from build123d import *

# Parameters (mm, degrees)
F0_W     = 16
F0_H     = 34
F1_DEPTH = 16
F2_W     = 10
F2_H     = 10
F3_DEPTH = 30
F4_W     = 10
F4_H     = 10
F5_DEPTH = 30
F6_R     = 1.5
F7_DEPTH = 16


with BuildPart() as f1:
    # F0 (on Top) → F1 (new body)
    with BuildSketch(Plane.XY):
        Polygon((25, 16), (-25, 16), (-25, 0), (-9, 0), (25, 0), align=None)
        with Locations((-17, -17)):
            Rectangle(F0_W, F0_H)
    extrude(amount=F1_DEPTH)

    # F2 (on face) → F3 (cut)
    with BuildSketch(Plane.YZ.offset(25)):
        with Locations((8, 8)):
            Rectangle(F2_W, F2_H)
    extrude(amount=-F3_DEPTH, mode=Mode.SUBTRACT)

    # F4 (on face) → F5 (cut)
    with BuildSketch(Plane.XZ.offset(34)):
        with Locations((-17, 8)):
            Rectangle(F4_W, F4_H)
    extrude(amount=-F5_DEPTH, mode=Mode.SUBTRACT)

    # F6 (on face) → F7 (cut)
    with BuildSketch(Plane.XY.offset(16)):
        with Locations((-17, -26)):
            Circle(F6_R)
        with Locations((17, 8)):
            Circle(F6_R)
    extrude(amount=-F7_DEPTH, mode=Mode.SUBTRACT)


solid = f1.part
Input: part model. Units: mm. Frame: model coordinates. A direction names the side the tool comes from. Round coordinates to 2 decimals unless told otherwise and drop trailing zeros. Loops run counter-clockwise (first coordinate to the right, second up) from the corner with the lowest first, then second, coordinate; pieces in that order, holes last. Notation, with made-up numbers: M 10,16 L 29,16 A35 cw 29,48 Z; hole C -2,-10 d5. An arc over 180 degrees is marked long. Answer as CSV lines item,"result". Start each with the question number.
(1) Section A-A, the plane y = 8. Output: boundary loops of the cut face in (x, z).
(2) First-contact query: pin 1 (8 mm diameter, centred on y = -15.5, z = 10.5, fed in from +X); pin 2 (3 mm diameter, centred on x = -19, z = 8.5, fed in from -Y); pin 3 (10 mm diameter, centred on x = -3, y = -9.5, fed in from -Z). Flat tips, straight axial feed; report the tip coordinate or a pass-through.
(3) Section C-C, the plane y = -26. Output: boundary loops of the cut face in (x, z).
(4) Line query: line 1 (X direction, y = -15.5, z = 6); line 2 (Z direction, x = -13, y = -24); line 3 (Y direction, x = -17, z = 1.95). Output: solid intervals per line, ascending. Write a range as [from, to].
(5) Reachability of faces 4 (the flat face through (-9, -17, 8)), 5 (the flat face through (10, 8, 3)), 6 (the flat face through (-12, -19, 8)) from +Z, -Z, +X, -X, +Y, -Y: full face, straight path, thin tool, end or side. Return the list, or none.
(6) Draft query along Z for faces 1 (the flat face through (10, 13, 8)), 2 (the flat face through (-6, 2, 0)), 3 (the cylindrical face through (-18.11, -24.99, 1.52)). Return one class per face: released by +Z, released by -Z, zero draft, split by the parting line, or undercut.
(7) Section D-D, the plane x = -0.5. Output: boundary loops of the cut face in (y, z).
(8) Section B-B, the plane x = -17. Output: boundary loops of the cut face in (y, z).
Values found:
1,outline,"M -25,0 L 15.5,0 L 15.5,3 L -5,3 L -5,13 L 15.5,13 L 15.5,16 L -25,16 Z; M 18.5,0 L 25,0 L 25,3 L 18.5,3 Z; M 18.5,13 L 25,13 L 25,16 L 18.5,16 Z"
2,pin 1,"stops at x = -9"
2,pin 2,"stops at y = -4"
2,pin 3,"passes through"
3,outline,"M -25,0 L -18.5,0 L -18.5,3 L -22,3 L -22,13 L -18.5,13 L -18.5,16 L -25,16 Z; M -15.5,0 L -9,0 L -9,16 L -15.5,16 L -15.5,13 L -12,13 L -12,3 L -15.5,3 Z"
4,line 1,"x = [-25, -22], [-12, -9]"
4,line 2,"z = [0, 3], [13, 16]"
4,line 3,"y = [-34, -27.5], [-24.5, 16]"
5,face 4,"+Z, -Z, +X, -Y"
5,face 5,"+X"
5,face 6,"-Y"
6,face 1,"undercut"
6,face 2,"released by -Z"
6,face 3,"zero draft"
7,outline,"M 0,0 L 16,0 L 16,16 L 0,16 Z; hole M 3,3 L 13,3 L 13,13 L 3,13 Z"
8,outline,"M -34,0 L -27.5,0 L -27.5,3 L -34,3 Z; M -34,13 L -27.5,13 L -27.5,16 L -34,16 Z; M -24.5,0 L 16,0 L 16,16 L -24.5,16 L -24.5,13 L -4,13 L -4,3 L -24.5,3 Z"
